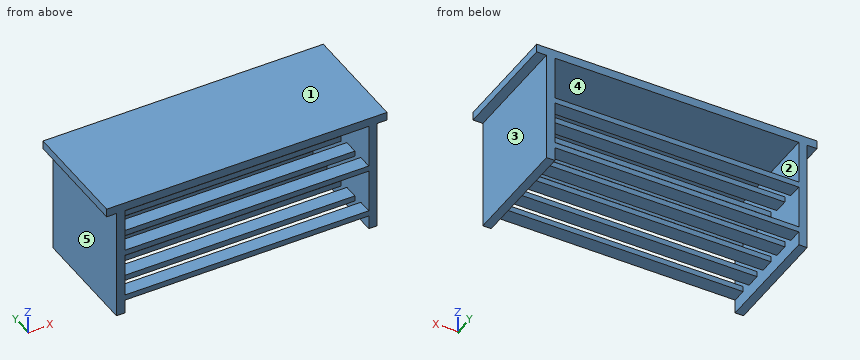
from build123d import *

# Parameters (mm, degrees)
F0_W     = 1000
F0_H     = 400
F1_DEPTH = 30
F2_W     = 30
F2_H     = 400
F3_DEPTH = 400
F4_W     = 50
F4_H     = 20
F5_DEPTH = 870


with BuildPart() as f1:
    # F0 (on Top) → F1 (new body)
    with BuildSketch(Plane.XY):
        Rectangle(F0_W, F0_H)
    extrude(amount=-F1_DEPTH)

    # F2 (on face) → F3 (join)
    with BuildSketch(Plane(origin=(0, 0, -30), x_dir=(1, 0, 0), z_dir=(0, 0, -1))):
        with Locations((-450, 0)):
            Rectangle(F2_W, F2_H)
        with Locations((450, 0)):
            Rectangle(F2_W, F2_H)
    extrude(amount=F3_DEPTH)

    # F4 (on face) → F5 (join, through all)
    with BuildSketch(Plane(origin=(435, 0, 0), x_dir=(0, -1, 0), z_dir=(-1, 0, 0))):
        with Locations((-175, -195)):
            Rectangle(F4_W, F4_H)
        with Locations((-87.5, -195)):
            Rectangle(F4_W, F4_H)
        with Locations((0, -195)):
            Rectangle(F4_W, F4_H)
        with Locations((87.5, -195)):
            Rectangle(F4_W, F4_H)
        with Locations((175, -195)):
            Rectangle(F4_W, F4_H)
        with Locations((175, -370)):
            Rectangle(F4_W, F4_H)
        with Locations((87.5, -370)):
            Rectangle(F4_W, F4_H)
        with Locations((0, -370)):
            Rectangle(F4_W, F4_H)
        with Locations((-87.5, -370)):
            Rectangle(F4_W, F4_H)
        with Locations((-175, -370)):
            Rectangle(F4_W, F4_H)
    extrude(amount=F5_DEPTH)


solid = f1.part
Verification items for the finished model (mm, model axes). Face numbers are marked on the shaded views. A direction names the side the tool comes from. Coordinates: 2 decimals unless noted, no trailing zeros. Write each loop counter-clockwise with the first axis right and the second up, starting at its lowest first coordinate (ties: lowest second). Pieces come first, ordered by that corner, then holes. Notation, with made-up numbers: (66, -23) - (100, -23) arc R16 ccw to (100, 2) - close; hole circle Ø10 at (76.5, -38.5). An arc over 180 degrees is marked (long way). Answer as a JSON object with one key per item and string values.
(1) Cross-section at A-A on y = -85.5. Record the cut outline in (x, z), plus the area to 3 significant figures.
Report:
{"outline": "(-500, -30) - (-465, -30) - (-465, -430) - (-435, -430) - (-435, -380) - (435, -380) - (435, -430) - (465, -430) - (465, -30) - (500, -30) - (500, 0) - (-500, 0) - close; hole (-435, -360) - (435, -360) - (435, -205) - (-435, -205) - close; hole (-435, -185) - (435, -185) - (435, -30) - (-435, -30) - close", "area": "88,800 mm^2"}
(2) Thickness scan on line 1 along Y through (x, z) = (-210.5, -203.5); line 2 along Z through (x, y) = (-232.5, -4.5); line 3 along X through (y, z) = (22.5, -65). Record the ranges inside material, lowest first.
Report:
{"line 1": "-200 to -150, -112.5 to -62.5, -25 to 25, 62.5 to 112.5, 150 to 200", "line 2": "-380 to -360, -205 to -185, -30 to 0", "line 3": "-465 to -435, 435 to 465"}
(3) Cross-section at B-B on z = -334.5. Record the cut outline in (x, y).
Report:
{"outline": "(-465, -200) - (-435, -200) - (-435, 200) - (-465, 200) - close; (435, -200) - (465, -200) - (465, 200) - (435, 200) - close"}
(4) Cross-section at C-C on x = -211.5. Give the number of separate pieces and of enclosed holes in the cut face, plus the area to 3 significant figures.
Report:
{"separate pieces": "11", "enclosed holes": "0", "area": "22,000 mm^2"}
(5) Tool access check on the marked faces 4 and 5. Record the directions out of +Z, -Z, +X, -X, +Y, -Y that give a thin tool (end or side, any length) a straight path to the whole face; none if there is none.
Report:
{"face 4": "+Y, -Y", "face 5": "-Z, -X, +Y, -Y"}
(6) Mould release check, pull along Z, two halves, no side actions. Record for the marked faces 1, 2 and 3: pulls with the +Z half, pulls with the -Z half, needs draft (parallel to the pull), parting line crosses it, or undercut.
Report:
{"face 1": "pulls with the +Z half", "face 2": "undercut", "face 3": "needs draft"}
(7) Gauge pin test, flat ends, axial feed: pin 1 Ø5 at (x, y) = (188.5, -40.5) entering from -Z; pin 2 Ø8 at (y, z) = (-56.5, -98.5) entering from +X; pin 3 Ø12 at (x, y) = (-255.5, -107) entering from -Z. Record the tip position at first contact, or that the pin passes through.
Report:
{"pin 1": "z = -30", "pin 2": "x = 465", "pin 3": "z = -380"}
